Can you work these out from the model? Positions are in its coordinate system, mm. A direction names the side the tool comes from. Give positions to 0.01 mm unless a question says otherwise; leave off trailing zeros. Loops run counter-clockwise (first coordinate to the right, second up) from the corner with the lowest first, then second, coordinate; pieces in that order, holes last. Notation, with made-up numbers: (50, 38.25) - (101, 38.25) arc R32 cw to (101, 69.25) - close; hole circle Ø5 at (72, 27). An arc over 180 degrees is marked (long way). Answer in a Markdown table with one row per item.
from build123d import *

# Parameters (mm, degrees)
F0_W     = 44.0846085548
F0_H     = 54.1256517172
F1_DEPTH = 12.7
F2_W     = 44.0846085548
F2_H     = 10.2772433311
F3_DEPTH = 63.5
F5_DEPTH = 10.16
F6_W     = 15.7867255621
F6_H     = 24.1755610228
F7_DEPTH = 10.2782433311


with BuildPart() as f1:
    # F0 (on Top) → F1 (new body)
    with BuildSketch(Plane.XY):
        with BuildLine():
            ThreePointArc((-22.0423042774, -27.0628258586), (0, -49.105130136), (22.0423042774, -27.0628258586))
            Line((22.0423042774, -27.0628258586), (-22.0423042774, -27.0628258586))
        make_face()
        Rectangle(F0_W, F0_H)
    extrude(amount=F1_DEPTH)

    # F2 (on face) → F3 (join)
    with BuildSketch(Plane.XY.offset(12.7)):
        with Locations((0, 21.9242041931)):
            Rectangle(F2_W, F2_H)
    extrude(amount=F3_DEPTH)

    # F4 (on face) → F5 (cut)
    with BuildSketch(Plane.YZ.offset(22.0423042774)):
        Polygon((16.7855825275, 12.7), (0, 12.7), (0, 0), (27.0628258586, 0), (27.0628258586, 26.5619661659), (16.7855825275, 26.5619661659), align=None)
    extrude(amount=-F5_DEPTH, mode=Mode.SUBTRACT)

    # F6 (on face) → F7 (cut, through all)
    with BuildSketch(Plane.XZ.offset(-16.7855825275)):
        with BuildLine():
            Line((4.5446627773, 52.0244389772), (-11.2420627847, 52.0244389772))
            ThreePointArc((-11.2420627847, 52.0244389772), (-3.3487000037, 44.1310761962), (4.5446627773, 52.0244389772))
        make_face()
        with Locations((-3.3487000037, 64.1122194886)):
            Rectangle(F6_W, F6_H)
    extrude(amount=-F7_DEPTH, mode=Mode.SUBTRACT)


solid = f1.part
Q1. Imagine slicing it at B-B, the plane x = 19. Write out the boundary of the cut face in (y, z), and give its area (3 significant figures).
Checked values:
| item | result |
|---|---|
| outline | (-38.24, 0) - (0, 0) - (0, 12.7) - (-38.24, 12.7) - close; (16.79, 26.56) - (27.06, 26.56) - (27.06, 76.2) - (16.79, 76.2) - close |
| area | 996 mm² |
Q2. Imagine slicing it at C-C, the plane z = 22.5. Write out the boundary of the cut face in (x, y).
Checked values:
| item | result |
|---|---|
| outline | (-22.04, 16.79) - (11.88, 16.79) - (11.88, 27.06) - (-22.04, 27.06) - close |
Q3. On a 3-axis mill with a long thin cutter (end or side, diameter ignored), from which of +Z, -Z, +X, -X, +Y, -Y can I reach the whole of each face in a straight line? I mean faces 5 (the face through (17, 0, 6)), 6 (the face through (11.882, 16, 11)), 7 (the face through (17, 22, 26.562)), 8 (the face through (0, 16.786, 44)). Say none if no direction works.
Checked values:
| item | result |
|---|---|
| face 5 | +Z, -Z, +X, +Y |
| face 6 | -Z, +X, +Y |
| face 7 | -Z, +X, +Y, -Y |
| face 8 | +Z, +X, -X, -Y |
Q4. If I drill on line 1 (X direction, y = 17.5, z = 65); line 2 (Z direction, x = 7.5, y = 13); line 3 (Y direction, x = 1, z = 21), over which ranges is the centre line in solid material (lowest first)? Write a range as [from, to].
Checked values:
| item | result |
|---|---|
| line 1 | x = [-22.04, -11.24], [4.54, 22.04] |
| line 2 | z = [0, 12.7] |
| line 3 | y = [16.79, 27.06] |
Q5. Imagine slicing it at D-D, the plane y = -7. Write out the boundary of the cut face in (x, z), and give its area (3 significant figures).
Checked values:
| item | result |
|---|---|
| outline | (-22.04, 0) - (22.04, 0) - (22.04, 12.7) - (-22.04, 12.7) - close |
| area | 560 mm² |
Q6. If we mould it in two halves opening along X, with no side actions, what happens to faces 1 (the face through (-3.522, 21.852, 44.133)), 2 (the face through (0, 27.063, 38)), 3 (the face through (4.545, 22, 64)), 4 (the face through (22.042, -14, 6))? For each: released by +X, released by -X, zero draft, split by the parting line, or undercut.
Checked values:
| item | result |
|---|---|
| face 1 | undercut |
| face 2 | zero draft |
| face 3 | undercut |
| face 4 | released by +X |
Q7. Imagine slicing it at A-A, the plane z = 65.5. Write out the boundary of the cut face in (x, y), and give its area (3 significant figures).
Checked values:
| item | result |
|---|---|
| outline | (-22.04, 16.79) - (-11.24, 16.79) - (-11.24, 27.06) - (-22.04, 27.06) - close; (4.54, 16.79) - (22.04, 16.79) - (22.04, 27.06) - (4.54, 27.06) - close |
| area | 291 mm² |
Q8. For pin 1 (8 mm diameter, centred on y = 9.5, z = 16.5, fed in from +X); pin 2 (22 mm diameter, centred on x = -5.5, y = -16, fed in from +Z), each with a flat end and sliding along its axis, tell me the tip position at first contact or that it passes through.
Checked values:
| item | result |
|---|---|
| pin 1 | stops at x = 11.88 |
| pin 2 | stops at z = 12.7 |
